The model under review builds one solid part; all positions refer to its coordinate system, in mm. Give positions to 0.01 mm unless a question says otherwise; leave off trailing zeros. Order: outer loops, then holes, each group sorted by start corner. A loop starts at its lowest first (then second) coordinate and runs counter-clockwise, first axis right, second up. Notation, with made-up numbers: (-11, -0.75) - (39, -0.75) arc R24 cw to (39, 10.25) - close; hole circle Ø1 at (62.25, 50.5). An arc over 180 degrees is marked (long way). Use CSV: the item, a comma, the result in double quotes. Start each with the question number.
1. To check wall thickness, follow line 1 (Y direction, x = 4.5, z = 42); line 2 (Z direction, x = -13, y = 19.5); line 3 (Z direction, x = 24, y = 30.5). State the ranges of each line that lie inside material, in increasing order. Write a range as [from, to].
2. For pin 1 (12 mm diameter, centred on x = -3.5, z = 56.5, fed in from -Y); pin 2 (1.5 mm diameter, centred on y = 2.5, z = 36, fed in from +X), all flat-tipped, find the tip position at first contact; note any pin that passes through.
3. Take a section at A-A, the plane x = 0. State the section outline as (y, z) points.
4. Draft analysis for pull direction Z (two halves, no side actions). For faces 1 (the flat face through (-1, 1, 0)), 2 (the cylindrical face through (-1.08, -4.88, 24.91)), 3 (the conical face through (-0.836, 6.365, 52.925)), 4 (the flat face through (0, 0, 90)), state which applies: released by +Z, released by -Z, zero draft, split by the parting line, or undercut.
5. Take a section at C-C, the plane z = 60.5. State the section outline as (x, y) points, then the cut area to 3 significant figures.
6. Take a section at B-B, the plane z = 32. State the section outline as (x, y) points, then the cut area to 3 significant figures.
```python
from build123d import *

# Parameters (mm, degrees)
F2_R      = 5
F3_DEPTH  = 80
F0_R      = 60
F3_FACE_R = 5
F8_R      = 5
F6_R      = 7.8


with BuildPart() as f3:
    # F2 (on offset) → F3 (new body)
    with BuildSketch(Plane.XY.offset(10)):
        Circle(F2_R)
    extrude(amount=F3_DEPTH)

    # F0 (on Top) → F4 section 0
    with BuildSketch(Plane.XY):
        Circle(F0_R)
    # F3_face (on face) → F4 section 1
    with BuildSketch(Plane(origin=(0, 0, 10), x_dir=(1, 0, 0), z_dir=(0, 0, -1))):
        Circle(F3_FACE_R)
    loft()

    # F8 (on offset) → F9 section 0
    with BuildSketch(Plane.XY.offset(40.25)):
        Circle(F8_R)
    # F6 (on offset) → F9 section 1
    with BuildSketch(Plane.XY.offset(65.25)):
        Circle(F6_R)
    loft()


solid = f3.part
```
Determined:
1,line 1,"y = [-2.6, 2.6]"
1,line 2,"z = [0, 6.65]"
1,line 3,"z = [0, 3.85]"
2,pin 1,"stops at y = -7.39"
2,pin 2,"stops at x = 4.68"
3,outline,"(-60, 0) - (60, 0) - (5, 10) - (5, 40.25) - (7.8, 65.25) - (5, 65.25) - (5, 90) - (-5, 90) - (-5, 65.25) - (-7.8, 65.25) - (-5, 40.25) - (-5, 10) - close"
4,face 1,"released by -Z"
4,face 2,"undercut"
4,face 3,"undercut"
4,face 4,"released by +Z"
5,outline,"circle Ø14.54 at (0, 0)"
5,area,"166 mm²"
6,outline,"circle Ø10 at (0, 0)"
6,area,"78.5 mm²"
